```python
from build123d import *

# Parameters (mm, degrees)
F0_W     = 44.45
F0_H     = 44.45
F1_DEPTH = 3.175
F2_R     = 5.08
F3_R     = 6.35
F4_DEPTH = 6.351


with BuildPart() as f1:
    # F0 (on Front) → F1 (new body, symmetric)
    with BuildSketch(Plane.XZ):
        Rectangle(F0_W, F0_H)
    extrude(amount=F1_DEPTH, both=True)

    # F2
    f2_edges = [f1.edges().sort_by_distance(p)[0] for p in [
        (-22.225, 0, 22.225),
        (22.225, 0, 22.225),
        (22.225, 0, -22.225),
        (-22.225, 0, -22.225),
    ]]
    fillet(f2_edges, radius=F2_R)

    # F3 (on face) → F4 (cut, through all)
    with BuildSketch(Plane.XZ.offset(3.175)):
        with Locations((-9.525, 9.525)):
            Circle(F3_R)
    extrude(amount=-F4_DEPTH, mode=Mode.SUBTRACT)


solid = f1.part
```
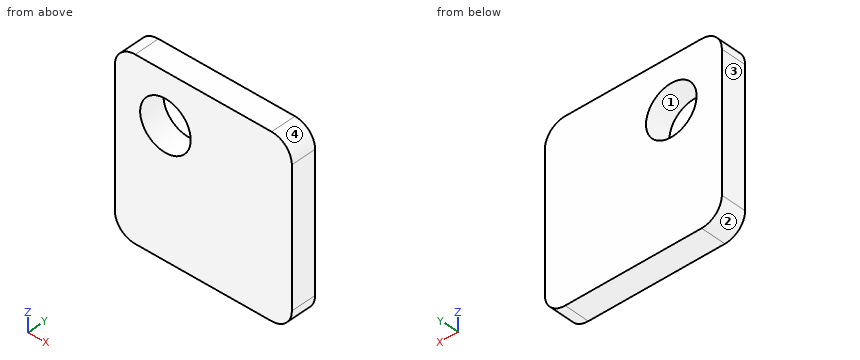
Geometry: final body of the model. Coordinates: model frame, mm. Face numbers are marked on the shaded views. Round coordinates to 2 decimals unless told otherwise and drop trailing zeros. Write each loop counter-clockwise with the first axis right and the second up, starting at its lowest first coordinate (ties: lowest second). Pieces come first, ordered by that corner, then holes. Notation, with made-up numbers: (12.25, 32) -> (16.25, 32) arc R21 cw to (16.25, 47) -> close; hole circle Ø2 at (23, 20). An arc over 180 degrees is marked (long way). Use CSV: the item, a comma, the result in double quotes. Start each with the question number.
Q1. Line query: L1, parallel to Z at x = -11, y = 0.75 (3 decimals); L2, parallel to X at y = 0, z = 11 (3 decimals); L3, parallel to Z at x = -6, y = 0.5 (3 decimals). Output: solid intervals per line, ascending.
Q2. Pull-direction query (Z, two-part tool) for the marked faces 1, 2, 3 and 4; classes: pulls with the +Z half, pulls with the -Z half, needs draft (parallel to the pull), parting line crosses it, or undercut.
Q3. Section A-A (x = -11.5). Return loops of the section in (y, z) (3 decimals), plus the area to 3 significant figures.
Q4. First-contact query: pin 1 Ø14.5 at (x, z) = (-9.525, 9.525) entering from -Y (3 decimals). Flat tip, straight axial feed; report the tip coordinate or a pass-through.
Q5. Section D-D (z = -19). Return loops of the section in (x, y) (3 decimals), plus the area to 3 significant figures.
Q6. Section C-C (y = 0). Return loops of the section in (x, z) (3 decimals).
Q7. Section B-B (z = 13.5). Return loops of the section in (x, y) (3 decimals), plus the area to 3 significant figures.
Result sheet:
1,L1,"-22.225 to 3.349, 15.701 to 22.225"
1,L2,"-22.225 to -15.701, -3.349 to 22.225"
1,L3,"-22.225 to 4.243, 14.807 to 22.225"
2,face 1,"undercut"
2,face 2,"pulls with the -Z half"
2,face 3,"needs draft"
2,face 4,"pulls with the +Z half"
3,outline,"(-3.175, -22.225) -> (3.175, -22.225) -> (3.175, 3.49) -> (-3.175, 3.49) -> close; (-3.175, 15.56) -> (3.175, 15.56) -> (3.175, 22.225) -> (-3.175, 22.225) -> close"
3,area,"206 mm²"
4,pin 1,"y = -3.175"
5,outline,"(-21.874, -3.175) -> (21.874, -3.175) -> (21.874, 3.175) -> (-21.874, 3.175) -> close"
5,area,"278 mm²"
6,outline,"(-22.225, -17.145) arc R5.08 ccw to (-17.145, -22.225) -> (17.145, -22.225) arc R5.08 ccw to (22.225, -17.145) -> (22.225, 17.145) arc R5.08 ccw to (17.145, 22.225) -> (-17.145, 22.225) arc R5.08 ccw to (-22.225, 17.145) -> close; hole circle Ø12.7 at (-9.525, 9.525)"
7,outline,"(-22.225, -3.175) -> (-14.477, -3.175) -> (-14.477, 3.175) -> (-22.225, 3.175) -> close; (-4.573, -3.175) -> (22.225, -3.175) -> (22.225, 3.175) -> (-4.573, 3.175) -> close"
7,area,"219 mm²"
